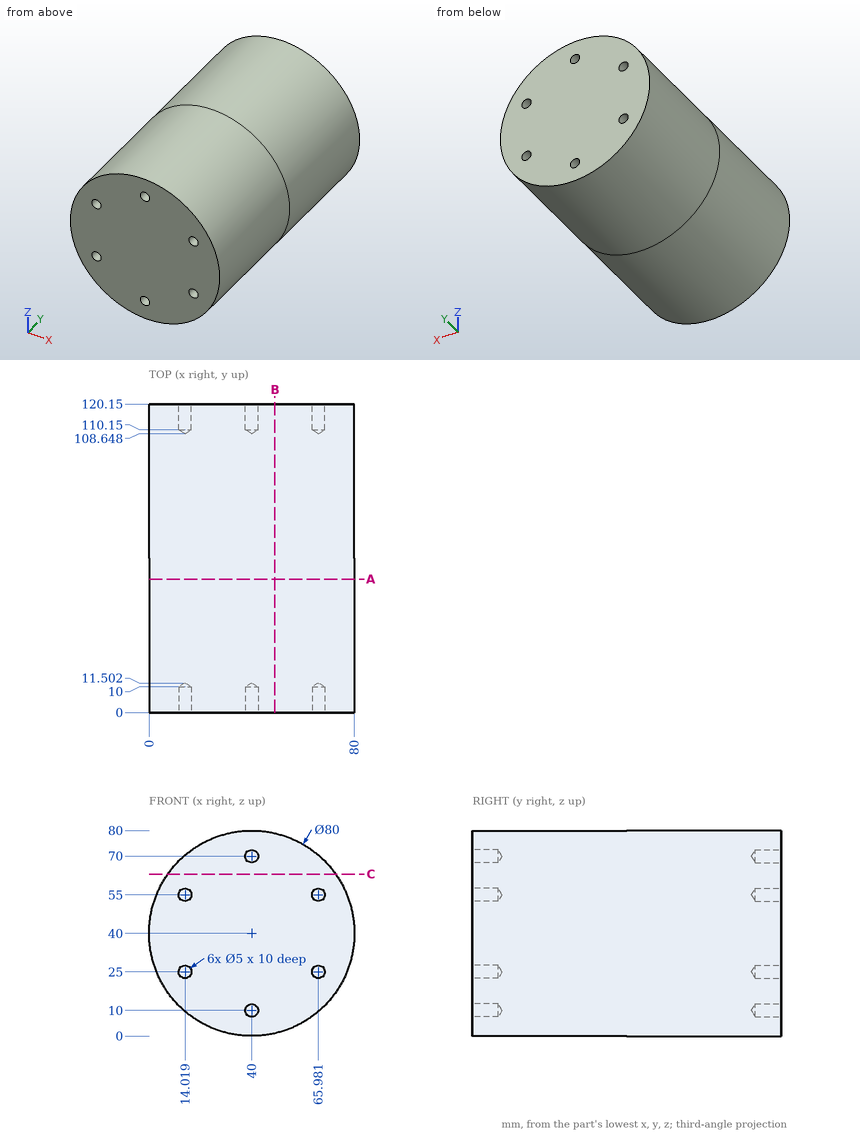
Geometry: see drawing. Coordinates: mm, zero at the bounding-box minimum. Give positions to 0.01 mm unless a question says otherwise; leave off trailing zeros. Order: outer loops, then holes, each group sorted by start corner. A loop starts at its lowest first (then second) coordinate and runs counter-clockwise, first axis right, second up.
Q1. Section A-A on y = 52. Output: boundary loops of the cut face in (x, z), and give its area (3 significant figures).
Checked values:
outline: circle Ø80 at (40, 40)
area: 5,030 mm2
Q2. Contact query for flat-ended pins moving along their axis: pin 1 Ø5 at (y, z) = (73, 60) entering from -X; pin 2 Ø12 at (y, z) = (36, 32) entering from +X; pin 3 Ø12 at (x, y) = (46.5, 93.5) entering from +Z. Output: stop coordinate, or through.
Checked values:
pin 1: stops at x = 4.03
pin 2: stops at x = 79.95
pin 3: stops at z = 80
Q3. Section C-C on z = 63. Output: boundary loops of the cut face in (x, y).
Checked values:
outline: (7.27, 0) - (72.73, 0) - (72.73, 120.15) - (7.27, 120.15) - close
Q4. Section B-B on x = 49. Output: boundary loops of the cut face in (y, z), and give its area (3 significant figures).
Checked values:
outline: (0, 1.03) - (120.15, 1.03) - (120.15, 78.97) - (0, 78.97) - close
area: 9,370 mm2
Q5. Ray query, probe 1 along X at (y, z) = (113, 24); probe 2 along X at (y, z) = (112.5, 25); probe 3 along Z at (x, y) = (42.5, 101). Return the intervals inside material, ascending.
Checked values:
probe 1: x = 3.34 to 11.73, 16.31 to 63.69, 68.27 to 76.66
probe 2: x = 2.92 to 11.52, 16.52 to 63.48, 68.48 to 77.08
probe 3: z = 0.08 to 79.92
